Verification items for the finished model (mm, model axes). A direction names the side the tool comes from. Give positions to 0.01 mm unless a question says otherwise; leave off trailing zeros. Write each loop counter-clockwise with the first axis right and the second up, starting at its lowest first coordinate (ties: lowest second). Pieces come first, ordered by that corner, then holes. Notation, with made-up numbers: (40.5, 36.25) - (61.5, 36.25) arc R18 cw to (61.5, 71.25) - close; hole circle Ø10 at (47, 69.25). An arc over 180 degrees is marked (long way). Put each result on its own line as item: value.
from build123d import *

# Parameters (mm, degrees)
CUT_EXTRUDE1_REACH      = 6
SKETCH13_R              = 1.5
SKETCH5_R               = 1.5
CUT_EXTRUDE2_DEPTH      = 13.5
CUT_EXTRUDE2_DEPTH_BACK = 13.5
CHAMFER1_SIZE           = 0.5


with BuildPart() as part:
    # Sketch1 → Revolve1 (revolve)
    with BuildSketch(Plane(origin=(0, 0, 0), x_dir=(1, 0, 0), z_dir=(0, 1, 0))):
        Polygon((0, 0), (0, 4), (4, 4), (4, 12), (5, 12), (5, 4), (12.5, 4), (12.5, 0), align=None)
    revolve(axis=Axis((0, 0, 0), (0, 0, 1)))

    # Sketch13 → Cut-Extrude1 (cut, up to next)
    with BuildSketch(Plane(origin=(0, 0, -4), x_dir=(-1, 0, 0), z_dir=(0, 0, -1)), mode=Mode.PRIVATE) as cut_extrude1_sk1:
        with Locations((-4.75, 8.227241336)):
            Circle(SKETCH13_R)
    cut_extrude1_tool1 = extrude(cut_extrude1_sk1.sketch, amount=-CUT_EXTRUDE1_REACH, mode=Mode.PRIVATE) & part.part
    add(cut_extrude1_tool1.solids().sort_by_distance((4.75, 8.227241, -4))[0], mode=Mode.SUBTRACT)
    # Sketch13 → Cut-Extrude1 (cut, up to next)
    with BuildSketch(Plane(origin=(0, 0, -4), x_dir=(-1, 0, 0), z_dir=(0, 0, -1)), mode=Mode.PRIVATE) as cut_extrude1_sk2:
        with Locations((-8.227241336, -4.75)):
            Circle(SKETCH13_R)
    cut_extrude1_tool2 = extrude(cut_extrude1_sk2.sketch, amount=-CUT_EXTRUDE1_REACH, mode=Mode.PRIVATE) & part.part
    add(cut_extrude1_tool2.solids().sort_by_distance((8.227241, -4.75, -4))[0], mode=Mode.SUBTRACT)
    # Sketch13 → Cut-Extrude1 (cut, up to next)
    with BuildSketch(Plane(origin=(0, 0, -4), x_dir=(-1, 0, 0), z_dir=(0, 0, -1)), mode=Mode.PRIVATE) as cut_extrude1_sk3:
        with Locations((4.75, -8.227241336)):
            Circle(SKETCH13_R)
    cut_extrude1_tool3 = extrude(cut_extrude1_sk3.sketch, amount=-CUT_EXTRUDE1_REACH, mode=Mode.PRIVATE) & part.part
    add(cut_extrude1_tool3.solids().sort_by_distance((-4.75, -8.227241, -4))[0], mode=Mode.SUBTRACT)
    # Sketch13 → Cut-Extrude1 (cut, up to next)
    with BuildSketch(Plane(origin=(0, 0, -4), x_dir=(-1, 0, 0), z_dir=(0, 0, -1)), mode=Mode.PRIVATE) as cut_extrude1_sk4:
        with Locations((8.227241336, 4.75)):
            Circle(SKETCH13_R)
    cut_extrude1_tool4 = extrude(cut_extrude1_sk4.sketch, amount=-CUT_EXTRUDE1_REACH, mode=Mode.PRIVATE) & part.part
    add(cut_extrude1_tool4.solids().sort_by_distance((-8.227241, 4.75, -4))[0], mode=Mode.SUBTRACT)

    # Sketch5 → Cut-Extrude2 (cut, two sides)
    with BuildSketch(Plane(origin=(0, 0, 0), x_dir=(0, 0, -1), z_dir=(1, 0, 0))) as cut_extrude2_sk:
        with Locations((8, 0)):
            Circle(SKETCH5_R)
    extrude(amount=CUT_EXTRUDE2_DEPTH, mode=Mode.SUBTRACT)
    extrude(cut_extrude2_sk.sketch, amount=-CUT_EXTRUDE2_DEPTH_BACK, mode=Mode.SUBTRACT)

    # Chamfer1
    chamfer1_edges = [part.edges().sort_by_distance(p)[0] for p in [
        (-5, 0, -12),
    ]]
    chamfer(chamfer1_edges, length=CHAMFER1_SIZE)


solid = part.part
Q1. Section check A-A, the plane y = 0. Record the cut outline in (x, z), plus the area to 3 significant figures.
Answers follow:
outline: (-12.5, -4) - (-5, -4) - (-5, -6.5) - (-4, -6.5) - (-4, -4) - (4, -4) - (4, -6.5) - (5, -6.5) - (5, -4) - (12.5, -4) - (12.5, 0) - (-12.5, 0) - close; (-5, -11.5) - (-4.5, -12) - (-4, -12) - (-4, -9.5) - (-5, -9.5) - close; (4, -12) - (4.5, -12) - (5, -11.5) - (5, -9.5) - (4, -9.5) - close
area: 110 mm2
Q2. Set-up check for faces 4 (the face through (-4.345, -1.464, -7.675)), 5 (the face through (0, 0, -4)): record each of +Z, -Z, +X, -X, +Y, -Y from which the full face is reachable in a straight line by a thin tool's end or side.
Answers follow:
face 4: +X, -X
face 5: -Z
Q3. Section check C-C, the plane z = -7.25. Record the cut outline in (x, y).
Answers follow:
outline: (-4.83, -1.3) arc R5 ccw to (4.83, -1.3) - (3.78, -1.3) arc R4 cw to (-3.78, -1.3) - close; (-4.83, 1.3) - (-3.78, 1.3) arc R4 cw to (3.78, 1.3) - (4.83, 1.3) arc R5 ccw to start
Q4. Section check D-D, the plane x = 0. Record the cut outline in (y, z), plus the area to 3 significant figures.
Answers follow:
outline: (-12.5, -4) - (-5, -4) - (-5, -11.5) - (-4.5, -12) - (-4, -12) - (-4, -4) - (4, -4) - (4, -12) - (4.5, -12) - (5, -11.5) - (5, -4) - (12.5, -4) - (12.5, 0) - (-12.5, 0) - close
area: 116 mm2
Q5. Go/stop test with flat-tipped pins: pin 1 Ø4 at (x, y) = (-8.23, 4.75) entering from -Z; pin 2 Ø3.5 at (y, z) = (0, -8) entering from +X; pin 3 Ø5 at (y, z) = (-7.5, -1.5) entering from +X; pin 4 Ø1 at (x, z) = (-0.5, -3.5) entering from +Y. Record where each tip stops, or that it passes through.
Answers follow:
pin 1: stops at z = -4
pin 2: stops at x = 5
pin 3: stops at x = 11.46
pin 4: stops at y = 12.5
Q6. Section check B-B, the plane x = -5.75. Record the cut outline in (y, z).
Answers follow:
outline: (-11.1, -4) - (-9.35, -4) - (-9.35, 0) - (-11.1, 0) - close; (-7.11, -4) - (11.1, -4) - (11.1, 0) - (-7.11, 0) - close
Q7. Scan lines: line 1 along X through (y, z) = (0.25, -10.75); line 2 along Z through (x, y) = (-9.5, -0.75); line 3 along Y through (x, z) = (0, -9.5). Record each from-to range of solid material in increasing order.
Answers follow:
line 1: x = -4.99 to -3.99, 3.99 to 4.99
line 2: z = -4 to 0
line 3: y = -5 to -4, 4 to 5
Q8. Release check for a two-part mould opening along Z. For faces 1 (the face through (4.345, -1.464, -7.675)), 2 (the face through (-5.556, -6.962, -2.028)), 3 (the face through (3, -3, -12)) record: released by +Z, released by -Z, zero draft, split by the parting line, or undercut.
Answers follow:
face 1: undercut
face 2: zero draft
face 3: released by -Z
